```python
from build123d import *

# Parameters (mm, degrees)
SKIZZE1_W                       = 10.1
SKIZZE1_H                       = 4.5
AUFSATZ_LINEAR_AUSTRAGEN1_DEPTH = 7.3
FASE2_SIZE                      = 1.8
AUFSATZ_LINEAR_AUSTRAGEN2_DEPTH = 0.255
LINEARES_MUSTER1_COUNT          = 2
LINEARES_MUSTER1_PITCH          = 2.54
LINEARES_MUSTER1_COL_COUNT      = 2
LINEARES_MUSTER1_COL_PITCH      = 2.54
VERRUNDUNG1_R                   = 0.1


with BuildPart() as part:
    # Skizze1 → Aufsatz-Linear austragen1 (new body)
    with BuildSketch(Plane(origin=(0, 0, 0), x_dir=(1, 0, 0), z_dir=(0, 1, 0))):
        Rectangle(SKIZZE1_W, SKIZZE1_H)
    extrude(amount=AUFSATZ_LINEAR_AUSTRAGEN1_DEPTH)

    # Fase2
    fase2_edges = [part.edges().sort_by_distance(p)[0] for p in [
        (5.05, 3.65, 2.25),
    ]]
    chamfer(fase2_edges, length=FASE2_SIZE)

    # Skizze3 → Aufsatz-Linear austragen2 (add, symmetric)
    with BuildSketch(Plane.XY.offset(-0.745)):
        Polygon((0, 0), (-0.698236912, 0), (-0.698236912, -1.502157044), (-0.349118456, -1.502157044), (-0.349118456, -10.505351049), (0.346596575, -10.505351049), (0.346596575, -1.502157044), (0.692124121, -1.502157044), (0.692124121, 0), align=None)
    aufsatz_linear_austragen2 = extrude(amount=AUFSATZ_LINEAR_AUSTRAGEN2_DEPTH, both=True)

    # Lineares Muster1: Aufsatz-Linear austragen2 ×2
    with Locations(*[(i * LINEARES_MUSTER1_PITCH, 0, 0) for i in range(1, LINEARES_MUSTER1_COUNT)]):
        add(aufsatz_linear_austragen2)

    # Lineares Muster1 col: Aufsatz-Linear austragen2 ×2
    with Locations(*[(-i * LINEARES_MUSTER1_COL_PITCH, 0, 0) for i in range(1, LINEARES_MUSTER1_COL_COUNT)]):
        add(aufsatz_linear_austragen2)

    # Verrundung1
    verrundung1_edges = [part.edges().sort_by_distance(p)[0] for p in [
        (-5.05, 7.3, 0),
        (-0.9, 7.3, 2.25),
        (5.05, 0, -0.9),
        (5.05, 7.3, -0.9),
        (5.05, 3.65, 0.45),
        (4.15, 0, 1.35),
        (3.25, 3.65, 2.25),
        (4.15, 7.3, 1.35),
        (0.692124121, 0, -0.745),
        (-0.698236912, 0, -0.745),
        (-0.003056396, 0, -1),
        (-0.003056396, 0, -0.49),
        (-1.847875879, 0, -0.745),
        (-0.9, 0, 2.25),
        (-3.238236912, 0, -0.745),
        (-2.543056396, 0, -1),
        (-2.543056396, 0, -0.49),
        (-5.05, 0, 0),
        (0, 0, -2.25),
        (3.232124121, 0, -0.745),
        (1.841763088, 0, -0.745),
        (2.536943604, 0, -1),
        (2.536943604, 0, -0.49),
        (0, 7.3, -2.25),
        (-5.05, 3.65, 2.25),
        (-5.05, 3.65, -2.25),
        (5.05, 3.65, -2.25),
    ]]
    fillet(verrundung1_edges, radius=VERRUNDUNG1_R)


solid = part.part
```
Here's how the part is built. I have some questions about the finished solid (model axes, mm). A direction names the side the tool comes from. Give positions to 0.01 mm unless a question says otherwise; leave off trailing zeros. Order: outer loops, then holes, each group sorted by start corner. A loop starts at its lowest first (then second) coordinate and runs counter-clockwise, first axis right, second up. Notation, with made-up numbers: (65.25, 21.25) - (70.25, 21.25) arc R4 cw to (70.25, 28.25) - close; hole circle Ø5 at (37.25, 22). An arc over 180 degrees is marked (long way). Answer as a JSON object with one key per item and string values. Group by question number.
Item 1: Please list where these lines run through material, in increasing order: probe 1 along Y at (x, z) = (2, 1.1); probe 2 along Z at (x, y) = (2.5, -8.75); probe 3 along X at (y, z) = (6, 0.55).
Item 2: Which directions (+Z, -Z, +X, -X, +Y, -Y) give clear straight access to the entire face, cutting with the end or side of a thin tool? Please do faces 1 (the flat face through (2.5, -5.2, -0.49)), 2 (the flat face through (0, -5, -1)), 3 (the flat face through (0, 4, -2.25)).
Item 3: If we section it at D-D on y = 4: Please give me the cut outline in (x, z).
Item 4: For P1, Ø1.5, axis at x = 0, y = -3, coming from the -Z side; P2, Ø0.6, axis at y = -0.5, z = -1, coming from the +X side; P3, Ø2, axis at x = 0, y = -7, coming from the +Z side; P4, Ø1.5, axis at y = -8, z = 1, coming from the -X side, each with a flat end and sliding along its axis, tell me the tip position at first contact or that it passes through.
Item 5: If we section it at C-C on x = -3.75: Please give me the cut outline in (y, z), and give its area (3 significant figures).
Item 6: If we section it at B-B on z = 0.05: Please give me the cut outline in (x, y).
Item 7: If we section it at A-A on y = -9.5: Please give me the cut outline in (x, z), and give its area (3 significant figures).
Result set:
{
 "1": {"probe 1": "0 to 7.3", "probe 2": "-1 to -0.49", "probe 3": "-5.05 to 4.95"},
 "2": {"face 1": "+Z, +X, -X, -Y", "face 2": "-Z, +X, -X, -Y", "face 3": "-Z, +X, -X, +Y, -Y"},
 "3": {"outline": "(-5.05, -2.15) arc R0.1 ccw to (-4.95, -2.25) - (4.95, -2.25) arc R0.1 ccw to (5.05, -2.15) - (5.05, 0.41) arc R0.1 ccw to (5.02, 0.48) - (3.28, 2.22) arc R0.1 ccw to (3.21, 2.25) - (-4.95, 2.25) arc R0.1 ccw to (-5.05, 2.15) - close"},
 "4": {"P1": "z = -1", "P2": "x = 3.23", "P3": "z = -0.49", "P4": "through"},
 "5": {"outline": "(0, -2.15) arc R0.1 ccw to (0.1, -2.25) - (7.2, -2.25) arc R0.1 ccw to (7.3, -2.15) - (7.3, 2.15) arc R0.1 ccw to (7.2, 2.25) - (0.1, 2.25) arc R0.1 ccw to (0, 2.15) - close", "area": "32.8 mm²"},
 "6": {"outline": "(-5.05, 0.1) arc R0.1 ccw to (-4.95, 0) - (4.95, 0) arc R0.1 ccw to (5.05, 0.1) - (5.05, 7.2) arc R0.1 ccw to (4.95, 7.3) - (-4.95, 7.3) arc R0.1 ccw to (-5.05, 7.2) - close"},
 "7": {"outline": "(-2.89, -1) - (-2.19, -1) - (-2.19, -0.49) - (-2.89, -0.49) - close; (-0.35, -1) - (0.35, -1) - (0.35, -0.49) - (-0.35, -0.49) - close; (2.19, -1) - (2.89, -1) - (2.89, -0.49) - (2.19, -0.49) - close", "area": "1.06 mm²"}
}
